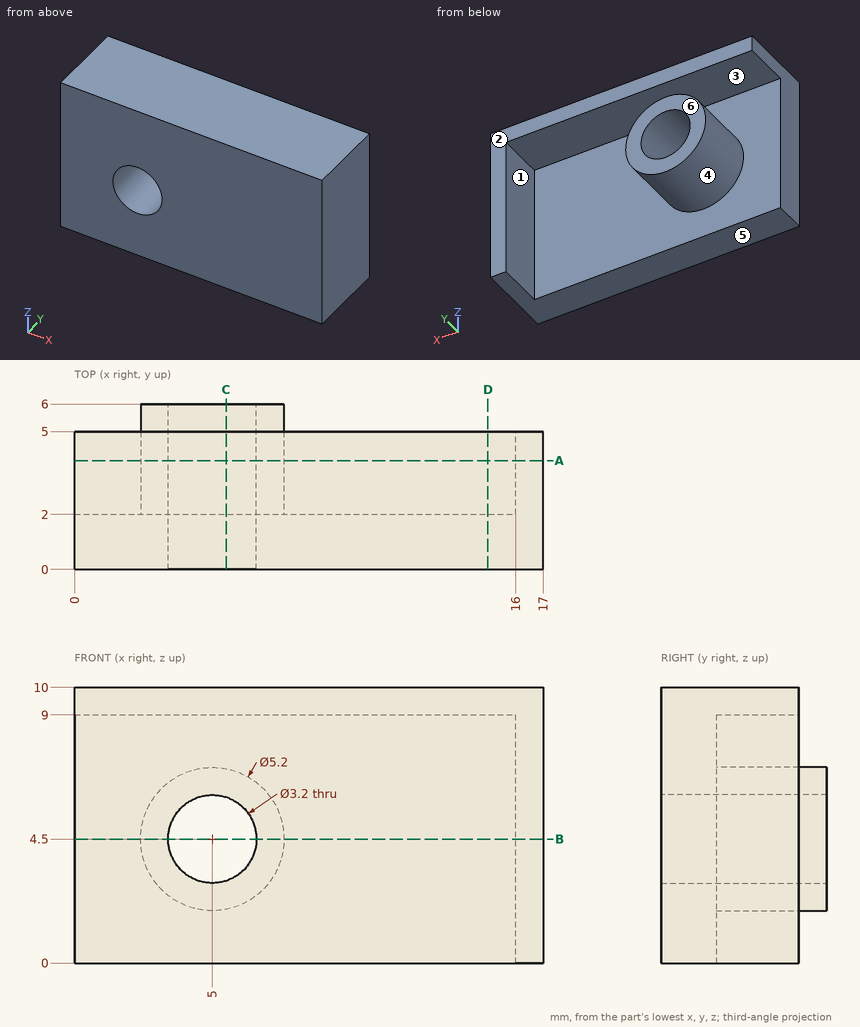
For this review, use the dimensioned drawing (mm, ordinates from the lowest corner) and the shaded views. A direction names the side the tool comes from. Round coordinates to 2 decimals unless told otherwise and drop trailing zeros. Write each loop counter-clockwise with the first axis right and the second up, starting at its lowest first coordinate (ties: lowest second). Pieces come first, ordered by that corner, then holes. Notation, with made-up numbers: M 28.5,-32 L 59.5,-32 A21 cw 59.5,-11 Z; hole C 73.25,50.25 d10. An arc over 180 degrees is marked long. Use CSV: the item, a comma, the result in double quotes. Start each with the question number.
(1) We need section A-A, the plane y = 3.95. State the section outline as (x, z) points.
(2) We need section D-D, the plane x = 15. State the section outline as (y, z) points.
(3) We need section B-B, the plane z = 4.5. State the section outline as (x, y) points.
(4) Tool access review of the marked faces 1, 2 and 3: name each direction out of +Z, -Z, +X, -X, +Y, -Y from which nothing blocks a thin tool from reaching the whole face with its end or side.
(5) We need section C-C, the plane x = 5.5. State the section outline as (y, z) points, then the cut area to 3 significant figures.
(6) Clearance check with flat-ended pins moving along their axes: P1, Ø1.5, axis at x = 11.5, y = 3.5, coming from the -Z side; P2, Ø6, axis at x = 14, z = 6.5, coming from the +Y side; P3, Ø0.9, axis at y = 3.5, z = 5, coming from the -X side. State where each tip first meets the part, or that it passes through.
(7) For line 1 along X through (y, z) = (4.05, 4.5); line 2 along X through (y, z) = (1.25, 4.5); line 3 along Z through (x, y) = (10.5, 3.75), list the stretches that pass through material, from the lowest coordinate up.
(8) The part is to be moulded in two halves that separate along Z. For the marked faces 4, 5 and 6, say which applies: +Z half, -Z half, draft (parallel to the pull), parting line (faces both ways), or undercut.
Findings:
1,outline,"M 0,9 L 16,9 L 16,0 L 17,0 L 17,10 L 0,10 Z; C 5,4.5 d5.2; hole C 5,4.5 d3.2"
2,outline,"M 0,0 L 2,0 L 2,9 L 5,9 L 5,10 L 0,10 Z"
3,outline,"M 0,0 L 3.4,0 L 3.4,6 L 2.4,6 L 2.4,2 L 0,2 Z; M 6.6,0 L 17,0 L 17,5 L 16,5 L 16,2 L 7.6,2 L 7.6,6 L 6.6,6 Z"
4,face 1,"-Z, +Y"
4,face 2,"+Z, +X, +Y"
4,face 3,"-X, +Y"
5,outline,"M 0,0 L 2,0 L 2,1.95 L 6,1.95 L 6,2.98 L 0,2.98 Z; M 0,6.02 L 6,6.02 L 6,7.05 L 2,7.05 L 2,9 L 5,9 L 5,10 L 0,10 Z"
5,area,"25.2 mm^2"
6,P1,"z = 9"
6,P2,"y = 5"
6,P3,"x = 2.4"
7,line 1,"2.4 to 3.4, 6.6 to 7.6, 16 to 17"
7,line 2,"0 to 3.4, 6.6 to 17"
7,line 3,"9 to 10"
8,face 4,"undercut"
8,face 5,"-Z half"
8,face 6,"draft"
